from build123d import *

# Parameters (mm, degrees)
SKETCH1_W           = 40
SKETCH1_H           = 3.9
BOSS_EXTRUDE1_DEPTH = 9
CUT_EXTRUDE1_REACH  = 24.276
SKETCH2_R           = 2.25
SKETCH3_W           = 0.75
SKETCH3_H           = 1.1
BOSS_EXTRUDE2_DEPTH = 9
FILLET1_R           = 0.1
CHAMFER1_SIZE       = 0.5


with BuildPart() as part:
    # Sketch1 → Boss-Extrude1 (new body)
    with BuildSketch(Plane.XY):
        with Locations((0, -1.95)):
            Rectangle(SKETCH1_W, SKETCH1_H)
    extrude(amount=BOSS_EXTRUDE1_DEPTH)

    # Sketch2 → Cut-Extrude1 (cut, up to next)
    with BuildSketch(Plane(origin=(0, 0, 0), x_dir=(1, 0, 0), z_dir=(0, 1, 0)), mode=Mode.PRIVATE) as cut_extrude1_sk1:
        with Locations(Location((0, -4.5, 0), (0, 0, 270))):
            Circle(SKETCH2_R)
    cut_extrude1_tool1 = extrude(cut_extrude1_sk1.sketch, amount=-CUT_EXTRUDE1_REACH, mode=Mode.PRIVATE) & part.part
    add(cut_extrude1_tool1.solids().sort_by_distance((0, 0, 4.5))[0], mode=Mode.SUBTRACT)

    # Sketch3 → Boss-Extrude2 (add)
    with BuildSketch(Plane.XY.offset(9)):
        with Locations((-17.625, 0.55)):
            Rectangle(SKETCH3_W, SKETCH3_H)
        with Locations((-19.625, 0.55)):
            Rectangle(SKETCH3_W, SKETCH3_H)
        with Locations((-15.625, 0.55)):
            Rectangle(SKETCH3_W, SKETCH3_H)
        with Locations((-13.625, 0.55)):
            Rectangle(SKETCH3_W, SKETCH3_H)
        with Locations((-11.625, 0.55)):
            Rectangle(SKETCH3_W, SKETCH3_H)
        with Locations((-9.625, 0.55)):
            Rectangle(SKETCH3_W, SKETCH3_H)
        with Locations((-7.625, 0.55)):
            Rectangle(SKETCH3_W, SKETCH3_H)
        with Locations((7.625, 0.55)):
            Rectangle(SKETCH3_W, SKETCH3_H)
        with Locations((9.625, 0.55)):
            Rectangle(SKETCH3_W, SKETCH3_H)
        with Locations((11.625, 0.55)):
            Rectangle(SKETCH3_W, SKETCH3_H)
        with Locations((13.625, 0.55)):
            Rectangle(SKETCH3_W, SKETCH3_H)
        with Locations((15.625, 0.55)):
            Rectangle(SKETCH3_W, SKETCH3_H)
        with Locations((17.625, 0.55)):
            Rectangle(SKETCH3_W, SKETCH3_H)
        with Locations((19.625, 0.55)):
            Rectangle(SKETCH3_W, SKETCH3_H)
    extrude(amount=-BOSS_EXTRUDE2_DEPTH)

    # Fillet1
    fillet1_edges = [part.edges().sort_by_distance(p)[0] for p in [
        (9.25, 1.1, 4.5),
        (10, 1.1, 4.5),
        (11.25, 1.1, 4.5),
        (12, 1.1, 4.5),
        (13.25, 1.1, 4.5),
        (14, 1.1, 4.5),
        (15.25, 1.1, 4.5),
        (16, 1.1, 4.5),
        (17.25, 1.1, 4.5),
        (18, 1.1, 4.5),
        (19.25, 1.1, 4.5),
        (20, 1.1, 4.5),
        (-20, 1.1, 4.5),
        (-19.25, 1.1, 4.5),
        (-18, 1.1, 4.5),
        (-17.25, 1.1, 4.5),
        (-16, 1.1, 4.5),
        (-15.25, 1.1, 4.5),
        (-14, 1.1, 4.5),
        (-13.25, 1.1, 4.5),
        (-12, 1.1, 4.5),
        (-11.25, 1.1, 4.5),
        (-10, 1.1, 4.5),
        (-9.25, 1.1, 4.5),
        (20, -3.9, 4.5),
        (-20, -3.9, 4.5),
        (-8, 1.1, 4.5),
        (-7.25, 1.1, 4.5),
        (7.25, 1.1, 4.5),
        (8, 1.1, 4.5),
    ]]
    fillet(fillet1_edges, radius=FILLET1_R)

    # Chamfer1
    chamfer1_edges = [part.edges().sort_by_distance(p)[0] for p in [
        (0, 0, 2.25),
    ]]
    chamfer(chamfer1_edges, length=CHAMFER1_SIZE)


solid = part.part
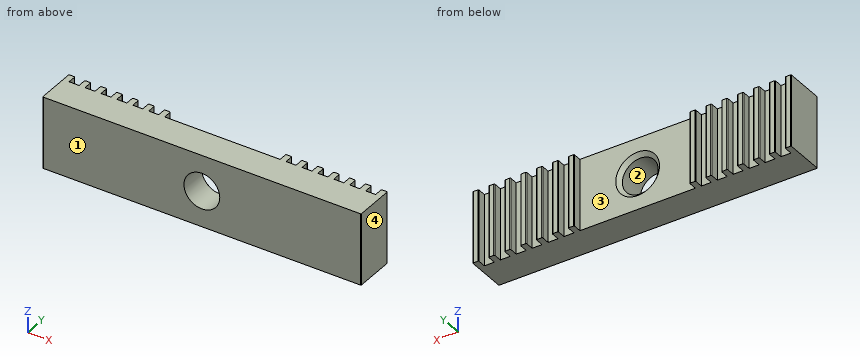
Work out the finished part from the listing and answer in its coordinate system (mm). Face numbers are marked on the shaded views. Give positions to 0.01 mm unless a question says otherwise; leave off trailing zeros. Loops run counter-clockwise (first coordinate to the right, second up) from the corner with the lowest first, then second, coordinate; pieces in that order, holes last. Notation, with made-up numbers: (-19, 71.5) - (27, 71.5) arc R26 cw to (27, 100.5) - close; hole circle Ø1 at (8.25, 32). An arc over 180 degrees is marked (long way). Answer in a Markdown table with one row per item. Add a question column.
Q1. The part is cut by section B-B (y = -2.9). Determine the outline of the cut face in (x, z), and give its area (3 significant figures).
Q2. The part is cut by section A-A (x = 0). Determine the outline of the cut face in (y, z).
Q3. Consider line 1 along X through (y, z) = (-2.2, 4.5); line 2 along Y through (x, z) = (11, 2.25); line 3 along X through (y, z) = (-0.6, 6). Determine where each line is inside the solid, lowest interval first.
Q4. Each of these flat-tipped pins is pushed along its axis until it touches: P1, Ø2, axis at x = 0.5, z = 5, coming from the -Y side; P2, Ø4, axis at x = 3, z = 1.5, coming from the +Y side; P3, Ø5, axis at x = 0, z = 4.5, coming from the +Y side. Where does it stop, or does it pass through?
Q5. Determine the mould class of the marked faces 1, 2, 3 and 4 for opening direction X: released by +X, released by -X, zero draft, split by the parting line, or undercut.
Solution:
| question | item | result |
|---|---|---|
| 1 | outline | (-20, 0) - (20, 0) - (20, 9) - (-20, 9) - close; hole circle Ø4.5 at (0, 4.5) |
| 1 | area | 344 mm² |
| 2 | outline | (-3.9, 0) - (0, 0) - (0, 1.75) - (-0.5, 2.25) - (-3.9, 2.25) - close; (-3.9, 6.75) - (-0.5, 6.75) - (0, 7.25) - (0, 9) - (-3.9, 9) - close |
| 3 | line 1 | x = -20 to -2.25, 2.25 to 20 |
| 3 | line 2 | y = -3.9 to 0 |
| 3 | line 3 | x = -20 to -1.68, 1.68 to 20 |
| 4 | P1 | passes through |
| 4 | P2 | stops at y = 0 |
| 4 | P3 | stops at y = -0.25 |
| 5 | face 1 | zero draft |
| 5 | face 2 | undercut |
| 5 | face 3 | undercut |
| 5 | face 4 | released by +X |
